CAD build for the part. Positions are in the model's coordinates, mm. Face numbers are marked on the shaded views. A direction names the side the tool comes from. Round coordinates to 2 decimals unless told otherwise and drop trailing zeros. Order: outer loops, then holes, each group sorted by start corner. A loop starts at its lowest first (then second) coordinate and runs counter-clockwise, first axis right, second up. Notation, with made-up numbers: (5, 55) - (63, 55) arc R20 ccw to (63, 80) - close; hole circle Ø4 at (-12, 42). An arc over 180 degrees is marked (long way). Write item = value, one per line.
from build123d import *

# Parameters (mm, degrees)
SKETCH1_R                = 31.75
BOSS_EXTRUDE1_DEPTH      = 82.55
SKETCH4_W                = 82.55
SKETCH4_H                = 19.05
BOSS_EXTRUDE2_DEPTH      = 46.99
BOSS_EXTRUDE2_DEPTH_BACK = 31.75
SKETCH5_W                = 82.55
SKETCH5_H                = 88.9
SKETCH5_R                = 15.875
BOSS_EXTRUDE3_DEPTH      = 19.05
CHAMFER1_SIZE            = 25.4
SKETCH8_W                = 82.55
SKETCH8_H                = 19.05
BOSS_EXTRUDE4_DEPTH      = 31.75
BOSS_EXTRUDE4_DEPTH_BACK = 50.8
SKETCH3_R                = 15.875
CUT_EXTRUDE2_DEPTH       = 163.576
SKETCH9_R                = 9.525
CUT_EXTRUDE3_DEPTH       = 163.576


with BuildPart() as part:
    # Sketch1 → Boss-Extrude1 (new body)
    with BuildSketch(Plane.XY):
        Circle(SKETCH1_R)
    extrude(amount=-BOSS_EXTRUDE1_DEPTH)

    # Sketch4 → Boss-Extrude2 (add, two sides)
    with BuildSketch(Plane(origin=(31.75, 0, 0), x_dir=(0, 0, -1), z_dir=(1, 0, 0))) as boss_extrude2_sk:
        with Locations((41.275, -22.225)):
            Rectangle(SKETCH4_W, SKETCH4_H)
    extrude(amount=BOSS_EXTRUDE2_DEPTH)
    extrude(boss_extrude2_sk.sketch, amount=-BOSS_EXTRUDE2_DEPTH_BACK)

    # Sketch5 → Boss-Extrude3 (add)
    with BuildSketch(Plane(origin=(78.74, 0, 0), x_dir=(0, 0, -1), z_dir=(1, 0, 0))):
        with Locations((41.275, 12.7)):
            Rectangle(SKETCH5_W, SKETCH5_H)
        with Locations((41.275, 31.75)):
            Circle(SKETCH5_R, mode=Mode.SUBTRACT)
    extrude(amount=BOSS_EXTRUDE3_DEPTH)

    # Chamfer1
    chamfer1_edges = [part.edges().sort_by_distance(p)[0] for p in [
        (88.265, 57.15, -82.55),
        (88.265, 57.15, 0),
    ]]
    chamfer(chamfer1_edges, length=CHAMFER1_SIZE)

    # Sketch8 → Boss-Extrude4 (add, two sides)
    with BuildSketch(Plane(origin=(-31.75, 0, 0), x_dir=(0, 0, -1), z_dir=(1, 0, 0))) as boss_extrude4_sk:
        with Locations((41.275, 22.225)):
            Rectangle(SKETCH8_W, SKETCH8_H)
    extrude(amount=BOSS_EXTRUDE4_DEPTH)
    extrude(boss_extrude4_sk.sketch, amount=-BOSS_EXTRUDE4_DEPTH_BACK)

    # Sketch3 → Cut-Extrude2 (cut)
    with BuildSketch(Plane.XY):
        Circle(SKETCH3_R)
    extrude(amount=-CUT_EXTRUDE2_DEPTH, mode=Mode.SUBTRACT)

    # Sketch9 → Cut-Extrude3 (cut)
    with BuildSketch(Plane(origin=(0, 31.75, 0), x_dir=(1, 0, 0), z_dir=(0, 1, 0))):
        with Locations((-57.15, 63.5)):
            Circle(SKETCH9_R)
        with Locations((-57.15, 19.05)):
            Circle(SKETCH9_R)
    extrude(amount=-CUT_EXTRUDE3_DEPTH, mode=Mode.SUBTRACT)


solid = part.part
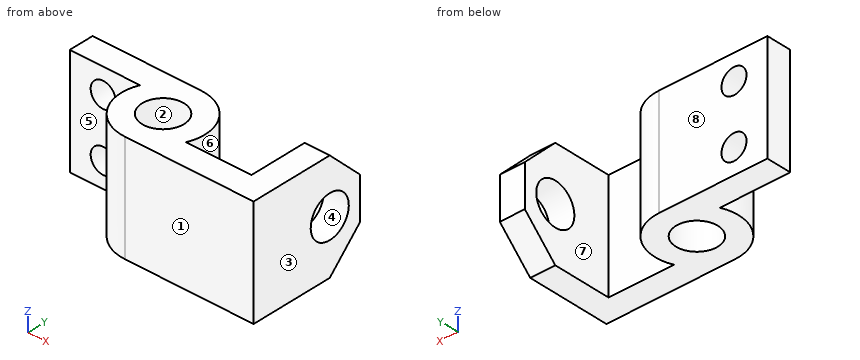
(1) Band-saw the part on C-C on x = 83.5. List the corners of the cut face in (y, z) (3 decimals).
Solved:
outline = (-31.75, -82.55) - (31.75, -82.55) - (57.15, -57.15) - (57.15, -25.4) - (31.75, 0) - (-31.75, 0) - close; hole circle Ø31.75 at (31.75, -41.275)
(2) Pull direction Y, two halves, no side cores. Call the marked faces 1, 2 and 3: released by +Y, released by -Y, zero draft, split by the parting line, or undercut.
Solved:
face_1 = released by -Y
face_2 = undercut
face_3 = zero draft
(3) Band-saw the part on A-A on z = -63.5. List the corners of the cut face in (x, y) (3 decimals), plus the area to 3 significant figures.
Solved:
outline = (-82.55, 12.7) - (-66.675, 12.7) - (-66.675, 31.75) - (-82.55, 31.75) - close; (-47.625, 12.7) - (-29.099, 12.7) arc R31.75 ccw to (0, -31.75) - (97.79, -31.75) - (97.79, 50.8) - (78.74, 50.8) - (78.74, -12.7) - (29.099, -12.7) arc R31.75 ccw to (0, 31.75) - (-47.625, 31.75) - close; hole circle Ø31.75 at (0, 0)
area = 5,860 mm²
(4) Probe line 1 along Z through (x, y) = (-57.15, 16.75) (3 decimals); line 2 along Y through (x, z) = (0, -21) (3 decimals); line 3 along Z through (x, y) = (91, 31). List the from-to ranges inside material, lowest first.
Solved:
line_1 = -82.55 to -73.025, -53.975 to -28.575, -9.525 to 0
line_2 = -31.75 to -15.875, 15.875 to 31.75
line_3 = -82.55 to -57.13, -25.42 to 0
(5) Band-saw the part on D-D on x = -57.15. List the corners of the cut face in (y, z) (3 decimals).
Solved:
outline = (12.7, -82.55) - (31.75, -82.55) - (31.75, -73.025) - (12.7, -73.025) - close; (12.7, -53.975) - (31.75, -53.975) - (31.75, -28.575) - (12.7, -28.575) - close; (12.7, -9.525) - (31.75, -9.525) - (31.75, 0) - (12.7, 0) - close
(6) Band-saw the part on B-B on y = 0. List the corners of the cut face in (x, z) (3 decimals).
Solved:
outline = (-31.75, -82.55) - (-15.875, -82.55) - (-15.875, 0) - (-31.75, 0) - close; (15.875, -82.55) - (31.75, -82.55) - (31.75, 0) - (15.875, 0) - close; (78.74, -82.55) - (97.79, -82.55) - (97.79, 0) - (78.74, 0) - close
(7) Tool access for the marked faces 4, 5, 6, 7 and 8: list every direction of +Z, -Z, +X, -X, +Y, -Y with a clear straight run to the whole face (end or side of a thin tool).
Solved:
face_4 = +X
face_5 = +Z, -Z, -X
face_6 = +Z, -Z
face_7 = +Z, -Z, +Y
face_8 = +Z, -Z, -X, +Y
(8) Drop flat-ended pins along their axis: pin 1 (10 mm diameter, centred on x = -53, z = -30, fed in from +Y); pin 2 (4 mm diameter, centred on x = -33.5, y = -11, fed in from +Z); pin 3 (16 mm diameter, centred on x = -64.5, z = -49.5, fed in from -Y). Give the stop position or say it passes through.
Solved:
pin_1 = 31.75
pin_2 = through
pin_3 = 12.7
